from build123d import *

# Parameters (mm, degrees)
BOSS_EXTRUDE2_DEPTH = 5


with BuildPart() as part:
    # Sketch3 → Boss-Extrude2 (new body)
    with BuildSketch(Plane.XY):
        with BuildLine():
            ThreePointArc((-18.75, 4.841229183), (-22.5, 0), (-18.75, -4.841229183))
            Line((-18.75, -4.841229183), (-9.375, -7.261843774))
            ThreePointArc((-9.375, -7.261843774), (0, 0), (-9.375, 7.261843774))
            Line((-9.375, 7.261843774), (-18.75, 4.841229183))
        make_face()
        with BuildLine():
            ThreePointArc((-12.082575695, 2), (-2.5, 0), (-12.082575695, -2))
            Line((-12.082575695, -2), (-14.72, -2))
            Line((-14.72, -2), (-14.72, 2))
            Line((-14.72, 2), (-12.082575695, 2))
        make_face(mode=Mode.SUBTRACT)
    extrude(amount=BOSS_EXTRUDE2_DEPTH)


solid = part.part
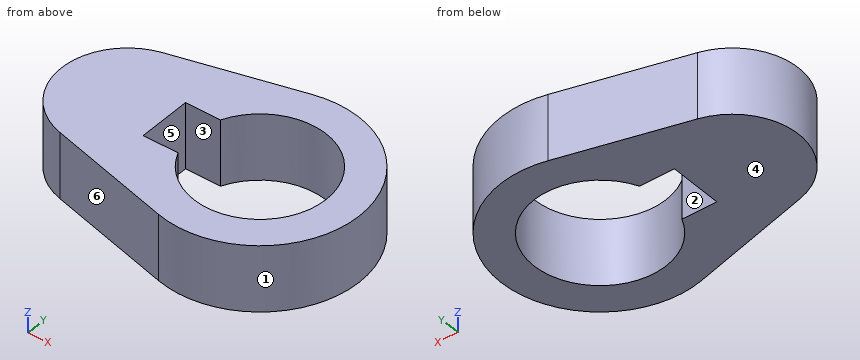
Geometry check sheet. Reference: the model listing, model coordinates, mm. Face numbers are marked on the shaded views. A direction names the side the tool comes from. Give positions to 0.01 mm unless a question says otherwise; leave off trailing zeros. Order: outer loops, then holes, each group sorted by start corner. A loop starts at its lowest first (then second) coordinate and runs counter-clockwise, first axis right, second up.
1) Cross-section at B-B (y = 0). Record the boundary of the cut face in (x, z), then the cut area to 3 significant figures.
Results are:
outline: (-22.5, 0) - (-14.72, 0) - (-14.72, 5) - (-22.5, 5) - close; (-2.5, 0) - (0, 0) - (0, 5) - (-2.5, 5) - close
area: 51.4 mm2
2) Material ranges on probe 1 along Y at (x, z) = (-7.5, 3.75); probe 2 along X at (y, z) = (2.25, 4.6); probe 3 along X at (y, z) = (-1, 2.85), recorded low to high.
Results are:
probe 1: y = -7.5 to -5, 5 to 7.5
probe 2: x = -21.97 to -11.97, -3.03 to -0.35
probe 3: x = -22.4 to -14.72, -2.6 to -0.07
3) Tool access check on the marked faces 5 and 6. Record the directions out of +Z, -Z, +X, -X, +Y, -Y that give a thin tool (end or side, any length) a straight path to the whole face; none if there is none.
Results are:
face 5: +Z, -Z
face 6: +Z, -Z, -X, -Y
4) Draft check along Y on the marked faces 1, 2, 3 and 4. Enter one of: released by +Y, released by -Y, zero draft, split by the parting line, or undercut.
Results are:
face 1: split by the parting line
face 2: undercut
face 3: undercut
face 4: zero draft
5) Cross-section at C-C (z = 3.25). Record the boundary of the cut face in (x, y) (3 decimals), then the cut area to 3 significant figures.
Results are:
outline: (-18.75, -4.841) - (-9.375, -7.262) arc R7.5 ccw (long way) to (-9.375, 7.262) - (-18.75, 4.841) arc R5 ccw to start; hole (-14.72, -2) - (-12.083, -2) arc R5 ccw (long way) to (-12.083, 2) - (-14.72, 2) - close
area: 169 mm2
6) Cross-section at D-D (x = -20.5). Record the boundary of the cut face in (y, z).
Results are:
outline: (-4, 0) - (4, 0) - (4, 5) - (-4, 5) - close
7) Gauge pin test, flat ends, axial feed: pin 1 (5 mm diameter, centred on x = -5.5, y = 6, fed in from -Z); pin 2 (3 mm diameter, centred on y = 2.5, z = 4.5, fed in from -X); pin 3 (1.5 mm diameter, centred on y = 2.5, z = 2.5, fed in from -X); pin 4 (3 mm diameter, centred on x = -13, z = 2.5, fed in from +Y). Record the tip position at first contact, or that the pin passes through.
Results are:
pin 1: stops at z = 0
pin 2: stops at x = -22.4
pin 3: stops at x = -22.18
pin 4: stops at y = 6.71
8) Cross-section at A-A (x = -7.5). Record the boundary of the cut face in (y, z), then the cut area to 3 significant figures.
Results are:
outline: (-7.5, 0) - (-5, 0) - (-5, 5) - (-7.5, 5) - close; (5, 0) - (7.5, 0) - (7.5, 5) - (5, 5) - close
area: 25.0 mm2
